For this review, use the dimensioned drawing (mm, ordinates from the lowest corner) and the shaded views. Give positions to 0.01 mm unless a question says otherwise; leave off trailing zeros. Loops run counter-clockwise (first coordinate to the right, second up) from the corner with the lowest first, then second, coordinate; pieces in that order, holes last. Notation, with made-up numbers: (10, 80.5) -> (61, 80.5) arc R13 ccw to (61, 98.5) -> close; hole circle Ø6 at (-9, 26). An arc over 180 degrees is marked (long way). Write each question's results on one line, items separated by ' | '. Start each with the question number.
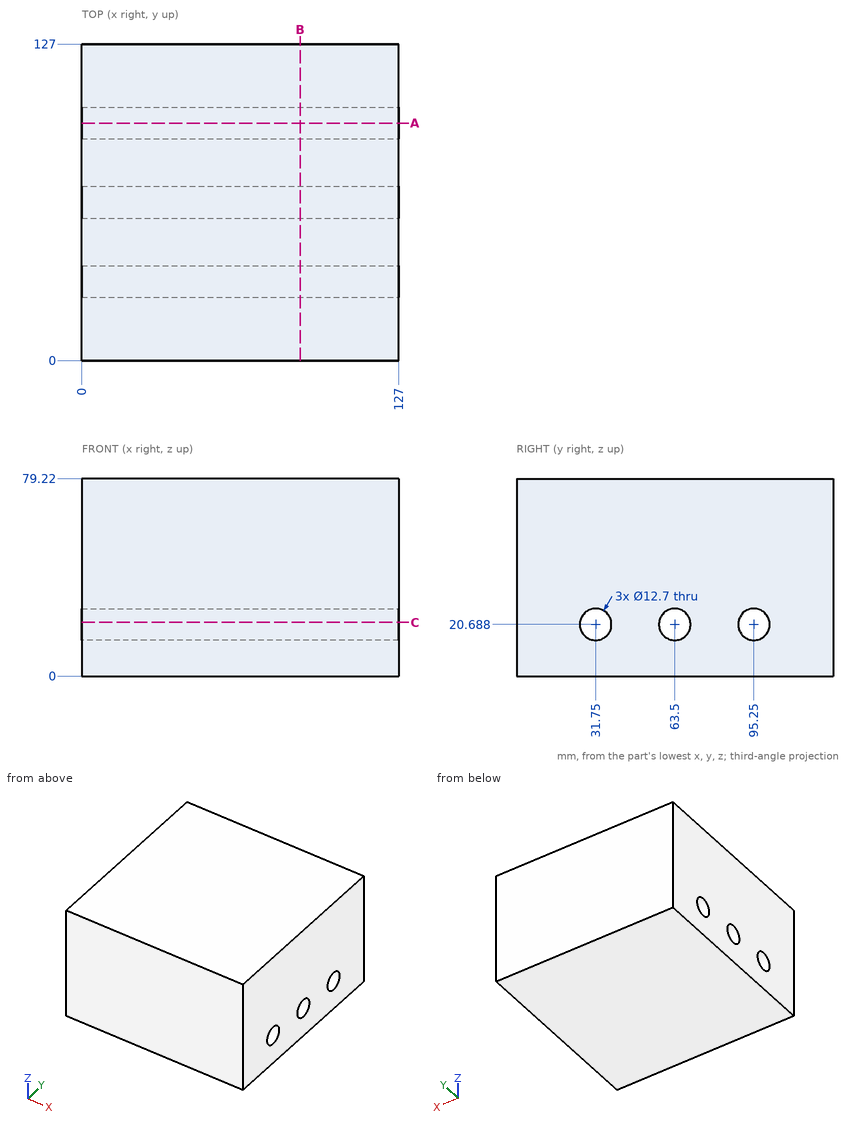
1. We need section A-A (y = 95.25). Write out the cut boundary in (x, z).
2. Wall thickness on L1, parallel to Z at x = 33, y = 95; L2, parallel to Y at x = 49, z = 19; L3, parallel to Y at x = 120.5, z = 16 (1 decimal): over which ranges is each line inside the solid? List them lowest first.
3. We need section B-B (x = 87.5). Write out the cut boundary in (y, z), plus the area to 3 significant figures.
4. We need section C-C (z = 21.5). Write out the cut boundary in (x, y), plus the area to 3 significant figures.
Response:
1) outline: (0, 0) -> (127, 0) -> (127, 14.34) -> (0, 14.34) -> close; (0, 27.04) -> (127, 27.04) -> (127, 79.22) -> (0, 79.22) -> close
2) L1: z = 0 to 14.34, 27.03 to 79.22 | L2: y = 0 to 25.63, 37.87 to 57.38, 69.62 to 89.13, 101.37 to 127 | L3: y = 0 to 27.5, 36 to 59.2, 67.8 to 91, 99.5 to 127
3) outline: (0, 0) -> (127, 0) -> (127, 79.22) -> (0, 79.22) -> close; hole circle Ø12.7 at (31.75, 20.69); hole circle Ø12.7 at (63.5, 20.69); hole circle Ø12.7 at (95.25, 20.69) | area: 9,680 mm2
4) outline: (0, 0) -> (127, 0) -> (127, 25.45) -> (0, 25.45) -> close; (0, 38.05) -> (127, 38.05) -> (127, 57.2) -> (0, 57.2) -> close; (0, 69.8) -> (127, 69.8) -> (127, 88.95) -> (0, 88.95) -> close; (0, 101.55) -> (127, 101.55) -> (127, 127) -> (0, 127) -> close | area: 11,300 mm2
